The model under review builds one solid part; all positions refer to its coordinate system, in mm. A direction names the side the tool comes from. Coordinates: 2 decimals unless noted, no trailing zeros. Write each loop counter-clockwise with the first axis right and the second up, starting at its lowest first coordinate (ties: lowest second). Pieces come first, ordered by that corner, then holes.
```python
from build123d import *

# Parameters (mm, degrees)
SKETCH2_R          = 3.75
CUT_EXTRUDE1_DEPTH = 133.664991614
FILLET1_R          = 2
CUT_EXTRUDE2_DEPTH = 151.069983674
CUT_EXTRUDE3_DEPTH = 151.069983674


with BuildPart() as part:
    # Sketch1 → Revolve1 (revolve)
    with BuildSketch(Plane(origin=(0, 0, 0), x_dir=(1, 0, 0), z_dir=(0, 1, 0)), mode=Mode.PRIVATE) as revolve1_sk:
        Polygon((0, 0), (139, 0), (139, 25), (120, 25), (120, 40), (91.5, 40), (89, 37.5), (50, 37.5), (47.5, 40), (19, 40), (19, 25), (0, 25), align=None)
    revolve(revolve1_sk.sketch.rotate(Axis((0, 0, 0), (1, 0, 0)), 180), axis=Axis((0, 0, 0), (1, 0, 0)))

    # Sketch2 → Cut-Extrude1 (cut, through all)
    with BuildSketch(Plane(origin=(120, 0, 0), x_dir=(0, 0, -1), z_dir=(1, 0, 0))):
        with Locations((-8.282209443, 30.909626441)):
            Circle(SKETCH2_R)
        with Locations((8.282209443, 30.909626441)):
            Circle(SKETCH2_R)
        with Locations((22.627416998, 22.627416998)):
            Circle(SKETCH2_R)
        with Locations((30.909626441, 8.282209443)):
            Circle(SKETCH2_R)
        with Locations((30.909626441, -8.282209443)):
            Circle(SKETCH2_R)
        with Locations((22.627416998, -22.627416998)):
            Circle(SKETCH2_R)
        with Locations((8.282209443, -30.909626441)):
            Circle(SKETCH2_R)
        with Locations((-8.282209443, -30.909626441)):
            Circle(SKETCH2_R)
        with Locations((-22.627416998, -22.627416998)):
            Circle(SKETCH2_R)
        with Locations((-30.909626441, -8.282209443)):
            Circle(SKETCH2_R)
        with Locations((-30.909626441, 8.282209443)):
            Circle(SKETCH2_R)
        with Locations((-22.627416998, 22.627416998)):
            Circle(SKETCH2_R)
    extrude(amount=-CUT_EXTRUDE1_DEPTH, mode=Mode.SUBTRACT)

    # Fillet1
    fillet1_edges = [part.edges().sort_by_distance(p)[0] for p in [
        (120, 0, -25),
        (19, 0, -25),
    ]]
    fillet(fillet1_edges, radius=FILLET1_R)

    # Sketch3 → Cut-Extrude2 (cut, through all)
    with BuildSketch(Plane.ZY):
        with BuildLine():
            Line((0, 0), (0, 40))
            ThreePointArc((0, 40), (28.284271247, 28.284271247), (40, 0))
            Line((40, 0), (0, 0))
        make_face()
    extrude(amount=-CUT_EXTRUDE2_DEPTH, mode=Mode.SUBTRACT)

    # Sketch5 → Cut-Extrude3 (cut, through all)
    with BuildSketch(Plane.XY):
        with BuildLine():
            Line((2.644904711, 25), (5.20944533, 10.45576741))
            Line((5.20944533, 10.45576741), (6.077686218, 5.531728645))
            ThreePointArc((6.077686218, 5.531728645), (21.306650015, 12.23263309), (31.720772546, 25.208360839))
            Line((31.720772546, 25.208360839), (27.189233611, 27.321452148))
            Line((27.189233611, 27.321452148), (19, 31.140154495))
            Line((19, 31.140154495), (19, 27))
            ThreePointArc((19, 27), (18.414213562, 25.585786438), (17, 25))
            Line((17, 25), (2.644904711, 25))
        make_face()
        with BuildLine():
            Line((30, 40), (19, 40))
            Line((19, 40), (19, 31.140154495))
            Line((19, 31.140154495), (27.189233611, 27.321452148))
            ThreePointArc((27.189233611, 27.321452148), (29.288880214, 33.506811582), (30, 40))
        make_face()
        with BuildLine():
            Line((0, 25), (0, 10))
            ThreePointArc((0, 10), (2.614672282, 10.114159057), (5.20944533, 10.45576741))
            Line((5.20944533, 10.45576741), (2.644904711, 25))
            Line((2.644904711, 25), (0, 25))
        make_face()
    extrude(amount=-CUT_EXTRUDE3_DEPTH, mode=Mode.SUBTRACT)


solid = part.part
```
Item 1: Machinability: for faces 5 (the face through (5.637, 8.028, -12.019)), 6 (the face through (84, 20, 0)), 7 (the face through (21, 12, -15)), which of the approach directions +Z, -Z, +X, -X, +Y, -Y give a long, thin tool a straight path to every point of the face, cutting with its end or side? Answer none if there is none.
Solved:
face 5: +Z, -Z, +Y
face 6: +Z, +X, -X, +Y
face 7: +Z, -Z
Item 2: Take a section at B-B, the plane x = 106.5. Count the separate pieces of the cut face and the enclosed holes in it, plus the area to 3 significant figures.
Solved:
separate pieces: 1
enclosed holes: 9
area: 3,370 mm2
Item 3: For pin 1 (10 mm diameter, centred on x = 64.5, y = 13, fed in from +Z); pin 2 (4 mm diameter, centred on x = 70, z = 17, fed in from -Y); pin 3 (12 mm diameter, centred on y = -22.63, z = -22.63, fed in from +X), all flat-tipped, find the tip position at first contact; note any pin that passes through.
Solved:
pin 1: stops at z = 0
pin 2: stops at y = -34.37
pin 3: stops at x = 120.27
Item 4: Mouldability with a two-part tool opening along Y and no side actions: class faces 1 (the face through (69, 0, 20)), 2 (the face through (70.207, -27.748, 6.266)), 3 (the face through (70.2, -20.1, 25.4)), 4 (the face through (105.55, -29.2, -27.34)) as pulls with the +Y half, pulls with the -Y half, needs draft (parallel to the pull), parting line crosses it, or undercut.
Solved:
face 1: pulls with the +Y half
face 2: undercut
face 3: undercut
face 4: parting line crosses it
Item 5: To check wall thickness, follow line 1 along Y through (x, z) = (31, -11); line 2 along Y through (x, z) = (105, -20); line 3 along Z through (x, y) = (69.5, -19.5). State the ranges of each line that lie inside material, in increasing order.
Solved:
line 1: y = -38.46 to -33.49, -28.33 to 23.75, 25.54 to 28.33, 33.49 to 38.46
line 2: y = -34.64 to -25.3, -19.95 to 19.95, 25.3 to 34.64
line 3: z = -32.03 to -24.7, -20.56 to 20.56, 24.7 to 32.03
Item 6: Take a section at A-A, the plane x = 24. Write out the cut boundary in (y, z).
Solved:
outline: (0, 0) - (0, 40) arc R40 ccw (long way) to (14.52, -37.27) - (14.52, 0) - close; hole circle Ø7.5 at (-30.91, -8.28); hole circle Ø7.5 at (-30.91, 8.28); hole circle Ø7.5 at (-22.63, -22.63); hole circle Ø7.5 at (-22.63, 22.63); hole circle Ø7.5 at (-8.28, -30.91); hole circle Ø7.5 at (-8.28, 30.91); hole circle Ø7.5 at (8.28, -30.91)
